Work out the finished part from the listing and answer in its coordinate system (mm). Round coordinates to 2 decimals unless told otherwise and drop trailing zeros. Order: outer loops, then holes, each group sorted by start corner. A loop starts at its lowest first (then second) coordinate and runs counter-clockwise, first axis right, second up. Notation, with made-up numbers: M -13.5,4 L 8.5,4 A21 ccw 8.5,12 Z; hole C -6,15.5 d9. An arc over 180 degrees is marked long. Answer as a JSON object with one key per item and string values. Group by question number.
from build123d import *

# Parameters (mm, degrees)
SKETCH1_R           = 3.175
BOSS_EXTRUDE1_DEPTH = 3.175


with BuildPart() as part:
    # Sketch1 → Boss-Extrude1 (new body)
    with BuildSketch(Plane.XY):
        with BuildLine():
            ThreePointArc((-18.347125171, 5.126938458), (-18.797583349, -3.090851056), (-15.739512715, -10.731739817))
            ThreePointArc((-15.739512715, -10.731739817), (-3.702112305, -5.159153466), (-5.126938458, -18.347125171))
            ThreePointArc((-5.126938458, -18.347125171), (3.090851056, -18.797583349), (10.731739817, -15.739512715))
            ThreePointArc((10.731739817, -15.739512715), (5.159153466, -3.702112305), (18.347125171, -5.126938458))
            ThreePointArc((18.347125171, -5.126938458), (18.797583349, 3.090851056), (15.739512715, 10.731739817))
            ThreePointArc((15.739512715, 10.731739817), (3.702112305, 5.159153466), (5.126938458, 18.347125171))
            ThreePointArc((5.126938458, 18.347125171), (-3.090851056, 18.797583349), (-10.731739817, 15.739512715))
            ThreePointArc((-10.731739817, 15.739512715), (-5.159153466, 3.702112305), (-18.347125171, 5.126938458))
        make_face()
        Circle(SKETCH1_R, mode=Mode.SUBTRACT)
    extrude(amount=BOSS_EXTRUDE1_DEPTH)


solid = part.part
Item 1: Find section D-D (x = -4.5). Give the vertices of the cut face in (y, z) (3 decimals).
Item 2: The mould has two halves that part along X. Classify faces 1 (the flat face through (4, 0, 0)), 2 (the cylindrical face through (-18.816, -2.976, 1.565)), 3 (the cylindrical face through (-5.03, 3.89, 1.57)): +X half, -X half, draft (parallel to the pull), parting line (faces both ways), or undercut.
Item 3: Each of these flat-tipped pins is pushed along its axis until it touches: pin 1 (10 mm diameter, centred on x = -3, y = -8, fed in from +Z) (3 decimals); pin 2 (1 mm diameter, centred on y = -13.5, z = 1.5, fed in from -X); pin 3 (1 mm diameter, centred on y = 1, z = 0.5, fed in from +X); pin 4 (1 mm diameter, centred on x = -5.5, z = 1.5, fed in from -Y). Where does it stop, or does it pass through?
Item 4: Find section A-A (z = 2.35). Give the vertices of the cut face in (x, y) (3 decimals).
Item 5: Find section B-B (y = 0). Give the vertices of the cut face in (x, z) (3 decimals), and give its area (3 significant figures).
Item 6: Consider L1, parallel to X at y = 2, z = 1.85; L2, parallel to Y at x = 2, z = 2.8; L3, parallel to Y at x = 0, z = 2.3 (3 decimals). Determine where each line is inside the solid, lowest interval first.
Responses:
{
 "1": {"outline": "M -18.511,0 L -18.042,0 L -18.042,3.175 L -18.511,3.175 Z; M -4.658,0 L 4.807,0 L 4.807,3.175 L -4.658,3.175 Z; M 11.482,0 L 18.511,0 L 18.511,3.175 L 11.482,3.175 Z"},
 "2": {"face 1": "draft", "face 2": "-X half", "face 3": "undercut"},
 "3": {"pin 1": "stops at z = 3.175", "pin 2": "stops at x = -1", "pin 3": "stops at x = 19.04", "pin 4": "stops at y = -18.38"},
 "4": {"outline": "M -18.347,5.127 A19.05 ccw -15.74,-10.732 A7.62 cw long -5.127,-18.347 A19.05 ccw 10.732,-15.74 A7.62 cw long 18.347,-5.127 A19.05 ccw 15.74,10.732 A7.62 cw long 5.127,18.347 A19.05 ccw -10.732,15.74 A7.62 cw long Z; hole C 0,0 d6.35"},
 "5": {"outline": "M -19.05,0 L -3.175,0 L -3.175,3.175 L -19.05,3.175 Z; M 3.175,0 L 19.05,0 L 19.05,3.175 L 3.175,3.175 Z", "area": "101 mm^2"},
 "6": {"L1": "x = -18.94 to -15.86, -6.84 to -2.47, 2.47 to 18.94", "L2": "y = -18.94 to -2.47, 2.47 to 6.84, 15.86 to 18.94", "L3": "y = -19.05 to -3.175, 3.175 to 19.05"}
}
